Autodesk Inventor part; units mm, degrees
ref_plane "Work Plane1" through (29, 0, 0) normal (0, -1, 0) x (1, 0, 0)
ref_plane "YZ Plane" through (0, 0, 0) normal (1, 0, 0) x (0, 1, 0)
ref_plane "XZ Plane" through (0, 0, 0) normal (0, 1, 0) x (-1, 0, 0)
sketch "Skizze1" plane through (0, 0, 0) normal (0, 0, 1) x (1, 0, 0)
  line L0 (-2.6667, 0) -> (55, 0)
  line L1 (55, 0) -> (55, 6)
  line L2 (55, 6) -> (19, 6)
  line L3 (19, 6) -> (17.9264, 6)
  line L4 (17.9264, 6) -> (0, 6)
  line L5 (0, 6) -> (0, 9)
  line L6 (0, 9) -> (-12, 9)
  line L7 (-12, 9) -> (-12, 5.7735)
  line L8 (-12, 5.7735) -> (-6, 5.7735)
  line L9 (-6, 5.7735) -> (-2.6667, 0)
  line L10 (-25.4, 0) -> (68.4, 0)
  line L11 (0, -1.8) -> (0, 10.8)
  line L12 (19, 6) -> (0, 6) construction
  dimension "d1" = 36
  dimension "d2" = 1.0736
  dimension "d3" = 12
  dimension "d4" = 6
  dimension "d5" = 60
  dimension "d6" = 12
  dimension "d7" = 12
  dimension "d8" = 11.547
  dimension "d9" = 18
  dimension "d26" = 55
revolve "Körper" add sketch "Skizze1" angle 360 about axis through (-2.6667, 0, 0) along (1, 0, 0)
sketch "Skizze2" plane through (-12, 0, 0) normal (-1, 0, 0) x (0, 0, 1)
  circle A0 centre (0, 0) radius 5.7735
  line L0 (0, -12.6) -> (0, 12.6)
  line L1 (-12.6, 0) -> (12.6, 0)
  line L2 (5.7735, 0) -> (2.8868, -5)
  line L3 (2.8868, -5) -> (-2.8868, -5)
  line L4 (-2.8868, -5) -> (-5.7735, 0)
  line L5 (-5.7735, 0) -> (-2.8868, 5)
  line L6 (-2.8868, 5) -> (2.8868, 5)
  line L7 (2.8868, 5) -> (5.7735, 0)
extrude "Loch" add sketch "Skizze2" against normal up to next contours L7 A0 | A0 L2 | L6 L0 A0 | A0 L0 L3 | L0 L6 A0 | A0 L3 L0 | L4 A0 | A0 L5
fillet "Rundung1" radius 1.2 1 edges at (-12, -9, 0)
thread "Gewinde"
chamfer "Fase1" distance 1.0735 distance2 1.0735 1 edges at (55, -6, 0) measured on face at (55, 1.497, 1.3262)
ref_plane "Work Plane1" through (29, 0, 0) normal (0, -1, 0) x (1, 0, 0)
fillet "Fillet2" radius 0.1 1 edges at (0, -6, 0)
equation "\"d1\" = GEL"
equation "\"d3\" = KOH"
equation "\"d4\" = INTI"
equation "\"d6\" = GD"
equation "\"d7\" = BDM"
equation "\"d8\" = 1.1547 * SW"
equation "\"d9\" = KOD"
equation "\"d26\" = NLG"
equation "\"d30\" = R"
equation "\"d17\" = RR"
equation "\"d13\" = GEL"
equation "\"d15\" = -0.5 * SPD + 0.5 * GD"
equation "\"d16\" = GUL"
equation "\"GD\" = 12"
equation "\"NLG\" = 55"
equation "\"GEL\" = 36"
equation "\"KOD\" = 18"
equation "\"KOH\" = 12"
equation "\"INTI\" = 6"
equation "\"GAL\" = 0.61345 * PTC"
equation "\"GUL\" = 0.61345 * PTC"
equation "\"BDM\" = NND"
equation "\"RR\" = 1.2"
equation "\"SPD\" = NND - 1.2269 * PTC"
equation "\"R\" = 0.1"
equation "\"TOA\" = 30deg"
equation "\"GD1\" = THREADDIA - 1.2269 * PTC"
equation "\"THREADDIA\" = 12"
equation "\"FAWI\" = 45deg"
equation "\"PTC\" = 1.75"
equation "\"NND\" = 12"
equation "\"E0\" = 1.155 * SW"
properties part number "ISO 4762 - M12 x 55" material "Edelstahl, 440C"
Here's how the part is built. I have some questions about the finished solid (model axes, mm). A direction names the side the tool comes from. Coordinates: 2 decimals unless noted, no trailing zeros. Order: outer loops, then holes, each group sorted by start corner. A loop starts at its lowest first (then second) coordinate and runs counter-clockwise, first axis right, second up. Notation, with made-up numbers: M 10,43.25 L 30,43.25 A15 cw 30,60.25 Z; hole C -35,85.5 d1. An arc over 180 degrees is marked long. Answer as CSV lines item,"result". Start each with the question number.
1. On a 3-axis mill with a long thin cutter (end or side, diameter ignored), from which of +Z, -Z, +X, -X, +Y, -Y can I reach the whole of each face in a straight line? I mean faces 5 (the flat face through (55, 0, 0)), 6 (the flat face through (-8.822, 2.535, 4.31)). Say none if no direction works.
2. We'd pull the mould along Y, two halves only. Please class faces 1 (the cylindrical face through (27, -6, 0)), 2 (the flat face through (-9, -5, 0)), 3 (the flat face through (-8.822, 2.465, -4.35)), 4 (the flat face through (0, 2, -6)): released by +Y, released by -Y, zero draft, split by the parting line, or undercut.
3. I need wall thicknesses on line 1 (X direction, y = 1.5, z = -7); line 2 (Y direction, x = 6, z = 0.25); line 3 (Y direction, x = -7.5, z = -4.25). Which ranges of each line are inside material? Lowest first, please. Write a range as [from, to].
4. I want a section at A-A, the plane x = 19.5. Write out the boundary of the cut face in (y, z).
5. For pin 1 (10 mm diameter, centred on x = -2.5, z = -0.5, fed in from -Y); pin 2 (3 mm diameter, centred on x = 27.5, y = 4, fed in from +Z); pin 3 (2 mm diameter, centred on x = 15.5, z = -4, fed in from -Y); pin 4 (2 mm diameter, centred on x = 25, y = -1, fed in from -Z), each with a flat end and sliding along its axis, tell me the tip position at first contact or that it passes through.
Recorded:
1,face 5,"+Z, -Z, +X, +Y, -Y"
1,face 6,"-X"
2,face 1,"split by the parting line"
2,face 2,"undercut"
2,face 3,"undercut"
2,face 4,"zero draft"
3,line 1,"x = [-12, 0]"
3,line 2,"y = [-5.99, 5.99]"
3,line 3,"y = [-7.93, -2.64], [2.64, 7.93]"
4,outline,"C 0,0 d12"
5,pin 1,"stops at y = -9"
5,pin 2,"stops at z = 5.45"
5,pin 3,"stops at y = -5.2"
5,pin 4,"stops at z = -6"
